from build123d import *

# Parameters (mm, degrees)
F0_R     = 15.875
F0_R_2   = 9.525
F1_DEPTH = 25.4
F2_R     = 28.672816
F2_R_2   = 15.580682
F3_DEPTH = 25.4
F4_R     = 16.011724
F4_R_2   = 9.452636
F5_DEPTH = 12.7
F6_R     = 3.81


with BuildPart() as f1:
    # F0 (on Top) → F1 (new body)
    with BuildSketch(Plane.XY):
        with BuildLine():
            Line((9.242882, 27.038856), (4.901954, 28.151403))
            ThreePointArc((4.901954, 28.151403), (-28.575, 0), (4.901954, -28.151403))
            Line((4.901954, -28.151403), (9.242882, -27.038856))
            ThreePointArc((9.242882, -27.038856), (23.244849, -16.619496), (28.575, 0))
            ThreePointArc((28.575, 0), (23.244849, 16.619496), (9.242882, 27.038856))
        make_face()
        Circle(F0_R, mode=Mode.SUBTRACT)
        with BuildLine():
            ThreePointArc((9.242882, 27.038856), (7.094261, 27.680356), (4.901954, 28.151403))
            Line((4.901954, 28.151403), (9.242882, 27.038856))
        make_face()
        with BuildLine():
            Line((9.242882, -27.038856), (4.901954, -28.151403))
            ThreePointArc((4.901954, -28.151403), (7.094261, -27.680356), (9.242882, -27.038856))
        make_face()
        with BuildLine():
            Line((54.741256, 15.377975), (9.242882, 27.038856))
            ThreePointArc((9.242882, 27.038856), (23.244849, 16.619496), (28.575, 0))
            Line((28.575, 0), (34.925, 0))
            ThreePointArc((34.925, 0), (41.06737, 12.541592), (54.741256, 15.377975))
        make_face()
        with BuildLine():
            ThreePointArc((28.575, 0), (23.244849, -16.619496), (9.242882, -27.038856))
            Line((9.242882, -27.038856), (54.741256, -15.377975))
            ThreePointArc((54.741256, -15.377975), (41.06737, -12.541592), (34.925, 0))
            Line((34.925, 0), (28.575, 0))
        make_face()
        with BuildLine():
            ThreePointArc((66.675, 0), (63.341592, 9.73263), (54.741256, 15.377975))
            ThreePointArc((54.741256, 15.377975), (41.06737, 12.541592), (34.925, 0))
            ThreePointArc((34.925, 0), (41.06737, -12.541592), (54.741256, -15.377975))
            ThreePointArc((54.741256, -15.377975), (63.341592, -9.73263), (66.675, 0))
        make_face()
        with Locations((50.8, 0)):
            Circle(F0_R_2, mode=Mode.SUBTRACT)
    extrude(amount=F1_DEPTH)

    # F2 (on face) → F3 (join)
    with BuildSketch(Plane.XY.offset(25.4)):
        Circle(F2_R)
        Circle(F2_R_2, mode=Mode.SUBTRACT)
    extrude(amount=F3_DEPTH)

    # F4 (on face) → F5 (cut)
    with BuildSketch(Plane.XY.offset(25.4)):
        with Locations((50.8, 0)):
            Circle(F4_R)
        with Locations((50.8, 0)):
            Circle(F4_R_2, mode=Mode.SUBTRACT)
    extrude(amount=-F5_DEPTH, mode=Mode.SUBTRACT)

    # F6
    f6_edges = [f1.edges().sort_by_distance(p)[0] for p in [
        (52.718644, -15.896355, 19.05),
        (52.718644, 15.896355, 19.05),
    ]]
    fillet(f6_edges, radius=F6_R)


solid = f1.part
Geometry check sheet. Reference: the model listing, model coordinates, mm. A direction names the side the tool comes from. Round coordinates to 2 decimals unless told otherwise and drop trailing zeros. Order: outer loops, then holes, each group sorted by start corner. A loop starts at its lowest first (then second) coordinate and runs counter-clockwise, first axis right, second up. Notation, with made-up numbers: (89.25, -30) - (136.25, -30) arc R27 cw to (136.25, 5) - close; hole circle Ø10 at (-14.75, 0.5). An arc over 180 degrees is marked (long way). One line per question, with ' | ' between items. Start each with the question number.
(1) Thickness scan on L1, parallel to Y at x = 0, z = 15.75 (3 decimals); L2, parallel to Z at x = 48, y = -12.5; L3, parallel to Z at x = 32.5, y = 13. Record the ranges inside material, lowest first. Write a range as [from, to].
(2) Access from +Z, -Z, +X, -X, +Y, -Y to the whole of each face (thin tool, end or side, straight path). Record for faces 1 (the cylindrical face through (7.125, 27.673, 12.522)), 2 (the cylindrical face through (-3.441, -15.497, 12.522)), 3 (the flat face through (47, 9, 12.7)).
(3) Sectioned sample at D-D on y = -11. Record the cut outline in (x, z).
(4) Sectioned sample at C-C on z = 24. Record the cut outline in (x, y) (3 decimals), and give its area (3 significant figures).
(5) Release check for a two-part mould opening along X. For faces 4 (the cylindrical face through (27.35, 8.61, 37.92)), 5 (the cylindrical face through (14.86, 4.68, 37.92)), 6 (the cylindrical face through (7.06, -27.69, 12.52)), 7 (the cylindrical face through (59.6, -3.65, 6.26)) record: released by +X, released by -X, zero draft, split by the parting line, or undercut.
(6) Sectioned sample at A-A on x = 0. Record the cut outline in (y, z) (3 decimals).
(7) Sectioned sample at B-B on z = 10.5. Record the cut outline in (x, y) (3 decimals), and give its area (3 significant figures).
(8) Depth check by flat-ended pin: pin 1 Ø9.5 at (x, y) = (43, 1) entering from +Z; pin 2 Ø10 at (y, z) = (-17.5, 20) entering from -X; pin 3 Ø8 at (x, z) = (-16, 8.5) entering from -Y; pin 4 Ø18.5 at (x, y) = (0, 0) entering from +Z. Enter the tip coordinate at first touch or a pass-through.
Conclusion:
1) L1: y = [-28.575, -15.875], [15.875, 28.575] | L2: z = [0, 12.7] | L3: z = [0, 25.4]
2) face 1: -Z, +X, +Y | face 2: -Z | face 3: +Z, +X
3) outline: (-26.48, 25.4) - (-26.37, 25.4) - (-26.37, 0) - (-11.45, 0) - (-11.45, 25.4) - (-11.03, 25.4) - (-11.03, 50.8) - (-26.48, 50.8) - close; (11.03, 25.4) - (11.45, 25.4) - (11.45, 0) - (62.25, 0) - (62.25, 12.7) - (39.16, 12.7) - (39.16, 25.4) - (26.48, 25.4) - (26.48, 50.8) - (11.03, 50.8) - close
4) outline: (4.902, -28.151) arc R28.575 ccw to (9.243, -27.039) - (39.507, -19.282) arc R3.81 ccw to (40.913, -12.595) arc R16.012 cw to (40.913, 12.595) arc R3.81 ccw to (39.507, 19.282) - (9.243, 27.039) arc R28.575 ccw to (4.902, 28.151) arc R28.575 ccw (long way) to start; hole circle Ø31.75 at (0, 0) | area: 2,370 mm2
5) face 4: split by the parting line | face 5: undercut | face 6: released by +X | face 7: undercut
6) outline: (-28.673, 25.4) - (-28.575, 25.4) - (-28.575, 0) - (-15.875, 0) - (-15.875, 25.4) - (-15.581, 25.4) - (-15.581, 50.8) - (-28.673, 50.8) - close; (15.581, 25.4) - (15.875, 25.4) - (15.875, 0) - (28.575, 0) - (28.575, 25.4) - (28.673, 25.4) - (28.673, 50.8) - (15.581, 50.8) - close
7) outline: (4.902, -28.151) arc R28.575 ccw to (9.243, -27.039) - (54.741, -15.378) arc R15.875 ccw to (54.741, 15.378) - (9.243, 27.039) arc R28.575 ccw to (4.902, 28.151) arc R28.575 ccw (long way) to start; hole circle Ø31.75 at (0, 0); hole circle Ø19.05 at (50.8, 0) | area: 2,930 mm2
8) pin 1: stops at z = 12.7 | pin 2: stops at x = -25.7 | pin 3: stops at y = -25.93 | pin 4: passes through
